Source: CAD feature listing. Evaluate the final solid. Frame: model axes, mm. Face numbers are marked on the shaded views. A direction names the side the tool comes from. Give positions to 0.01 mm unless a question says otherwise; leave off trailing zeros. Loops run counter-clockwise (first coordinate to the right, second up) from the corner with the lowest first, then second, coordinate; pieces in that order, holes last. Notation, with made-up numbers: M -21.75,10.25 L -4.75,10.25 A27 cw -4.75,29.25 Z; hole C 28.5,-38 d10. An arc over 180 degrees is marked long. Answer in a Markdown table with one row per item.
```python
from build123d import *
from OCP.BRepFilletAPI import BRepFilletAPI_MakeChamfer

# Parameters (mm, degrees)
SKETCH1_W           = 45.5
SKETCH1_H           = 9.1
BOSS_EXTRUDE1_DEPTH = 7
SKETCH2_W           = 37.1
SKETCH2_H           = 2.85
CUT_EXTRUDE1_DEPTH  = 5
SKETCH3_R           = 0.8
CUT_EXTRUDE2_DEPTH  = 5
FILLET1_R           = 1
SKETCH4_W           = 0.75
SKETCH4_H           = 0.75
BOSS_EXTRUDE2_DEPTH = 6
SKETCH5_W           = 6
SKETCH5_H           = 2
BOSS_EXTRUDE3_DEPTH = 19.5
CUT_EXTRUDE3_REACH  = 33.79
SKETCH6_W           = 3.3
SKETCH6_H           = 4.4
CHAMFER1_SIZE       = 0.25
CHAMFER1_SIZE2      = 3.575166564


with BuildPart() as part:
    # Sketch1 → Boss-Extrude1 (new body)
    with BuildSketch(Plane(origin=(0, 0, 0), x_dir=(1, 0, 0), z_dir=(0, 1, 0))):
        Rectangle(SKETCH1_W, SKETCH1_H)
    extrude(amount=BOSS_EXTRUDE1_DEPTH)

    # Sketch2 → Cut-Extrude1 (cut)
    with BuildSketch(Plane(origin=(0, 7, 0), x_dir=(1, 0, 0), z_dir=(0, 1, 0))):
        Rectangle(SKETCH2_W, SKETCH2_H)
    extrude(amount=-CUT_EXTRUDE1_DEPTH, mode=Mode.SUBTRACT)

    # Sketch3 → Cut-Extrude2 (cut)
    with BuildSketch(Plane(origin=(0, 7, 0), x_dir=(1, 0, 0), z_dir=(0, 1, 0))):
        with Locations(Location((-20.65, 0, 0), (0, 0, 270))):
            Circle(SKETCH3_R)
    extrude(amount=-CUT_EXTRUDE2_DEPTH, mode=Mode.SUBTRACT)

    # Fillet1
    fillet1_edges = [part.edges().sort_by_distance(p)[0] for p in [
        (-22.75, 7, 0),
        (0, 7, 4.55),
        (22.75, 7, 0),
        (0, 7, -4.55),
    ]]
    fillet(fillet1_edges, radius=FILLET1_R)

    # Sketch4 → Boss-Extrude2 (add)
    with BuildSketch(Plane.XZ):
        with Locations((-21.75, 2.73)):
            Rectangle(SKETCH4_W, SKETCH4_H)
        with Locations((-21.75, 0.91)):
            Rectangle(SKETCH4_W, SKETCH4_H)
        with Locations((-21.75, -0.91)):
            Rectangle(SKETCH4_W, SKETCH4_H)
        with Locations((-21.75, -2.73)):
            Rectangle(SKETCH4_W, SKETCH4_H)
    boss_extrude2 = extrude(amount=BOSS_EXTRUDE2_DEPTH)

    # Mirror1: Boss-Extrude2 across plane
    add(boss_extrude2.mirror(Plane(origin=(0, 0, 0), x_dir=(0, 0, 1), z_dir=(1, 0, 0))))

    # Sketch5 → Boss-Extrude3 (add)
    with BuildSketch(Plane(origin=(0, 2, 0), x_dir=(1, 0, 0), z_dir=(0, 1, 0))):
        Rectangle(SKETCH5_W, SKETCH5_H)
    extrude(amount=BOSS_EXTRUDE3_DEPTH)

    # Sketch6 → Cut-Extrude3 (cut, up to next)
    with BuildSketch(Plane.XY.offset(1), mode=Mode.PRIVATE) as cut_extrude3_sk1:
        with Locations((0, 19.3)):
            Rectangle(SKETCH6_W, SKETCH6_H)
    cut_extrude3_tool1 = extrude(cut_extrude3_sk1.sketch, amount=-CUT_EXTRUDE3_REACH, mode=Mode.PRIVATE) & part.part
    add(cut_extrude3_tool1.solids().sort_by_distance((0, 19.3, 1))[0], mode=Mode.SUBTRACT)

    # Chamfer1: one chamfer whose edges measure the first distance from different faces: ONE call of the kernel's chamfer builder (chamfer() names one face for all edges)
    chamfer1_edges_1 = [part.edges().sort_by_distance(p)[0] for p in [
        (-3, 21.5, 0),
    ]]
    chamfer1_side_1 = [part.faces().sort_by_distance(p)[0] for p in [
        (-2.325, 21.5, 0),
    ]]
    chamfer1_edges_2 = [part.edges().sort_by_distance(p)[0] for p in [
        (3, 21.5, 0),
    ]]
    chamfer1_side_2 = [part.faces().sort_by_distance(p)[0] for p in [
        (2.325, 21.5, 0),
    ]]
    chamfer1 = BRepFilletAPI_MakeChamfer(part.part.solid().wrapped)
    for e in chamfer1_edges_1:
        chamfer1.Add(CHAMFER1_SIZE, CHAMFER1_SIZE2, e.wrapped, chamfer1_side_1[0].wrapped)  # the first distance lies on this face
    for e in chamfer1_edges_2:
        chamfer1.Add(CHAMFER1_SIZE, CHAMFER1_SIZE2, e.wrapped, chamfer1_side_2[0].wrapped)  # the first distance lies on this face
    add(Compound.cast(chamfer1.Shape()), mode=Mode.REPLACE)


solid = part.part
```
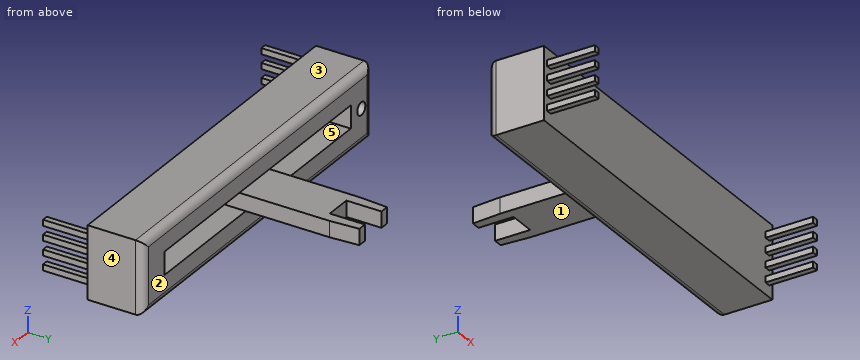
Q1. Reachability of the marked faces 4 and 5 from +Z, -Z, +X, -X, +Y, -Y: full face, straight path, thin tool, end or side. Return the list, or none.
Values follow:
| item | result |
|---|---|
| face 4 | +Z, -Z, +X, +Y, -Y |
| face 5 | +Y |
Q2. Mould query, pull axis Z, two halves, no side actions, for the marked faces 1, 2 and 3. Classes: +Z half, -Z half, draft (parallel to the pull), parting line (faces both ways), or undercut.
Values follow:
| item | result |
|---|---|
| face 1 | undercut |
| face 2 | draft |
| face 3 | +Z half |
Q3. Section query A-A (y = 5.5). Output: boundary loops of the cut face in (x, z) (3 decimals).
Values follow:
| item | result |
|---|---|
| outline | M -22.75,-4.55 L 22.75,-4.55 L 22.75,4.55 L -22.75,4.55 Z; M -3,-1 L 3,-1 L 3,1 L -3,1 Z; hole C -20.65,0 d1.6; hole M -18.55,-1.425 L 18.55,-1.425 L 18.55,1.425 L -18.55,1.425 Z |
Q4. Section query B-B (y = -3.25). Give the number of separate pieces and of enclosed holes in the cut face, plus the area to 3 significant figures.
Values follow:
| item | result |
|---|---|
| separate pieces | 8 |
| enclosed holes | 0 |
| area | 4.50 mm^2 |
Q5. Contact query for flat-ended pins moving along their axis: pin 1 Ø1.5 at (x, y) = (-1, 10) entering from +Z; pin 2 Ø4 at (x, z) = (13, -3) entering from -Y; pin 3 Ø0.8 at (y, z) = (-2, -3) entering from -X (3 decimals). Output: stop coordinate, or through.
Values follow:
| item | result |
|---|---|
| pin 1 | z = 1 |
| pin 2 | y = 0 |
| pin 3 | x = -22.125 |
Q6. Section query C-C (x = -20.65). Output: boundary loops of the cut face in (y, z).
Values follow:
| item | result |
|---|---|
| outline | M 0,-4.55 L 6,-4.55 A1 ccw 7,-3.55 L 7,-0.8 L 2,-0.8 L 2,0.8 L 7,0.8 L 7,3.55 A1 ccw 6,4.55 L 0,4.55 Z |
Q7. Section query D-D (z = 0). Output: boundary loops of the cut face in (x, y), plus the area to 3 significant figures.
Values follow:
| item | result |
|---|---|
| outline | M -22.75,0 L 22.75,0 L 22.75,6 A1 ccw 21.75,7 L 18.55,7 L 18.55,2 L 3,2 L 3,17.92 L 2.75,21.5 L 1.65,21.5 L 1.65,17.1 L -1.65,17.1 L -1.65,21.5 L -2.75,21.5 L -3,17.92 L -3,2 L -18.55,2 L -18.55,7 L -19.85,7 L -19.85,2 L -21.45,2 L -21.45,7 L -21.75,7 A1 ccw -22.75,6 Z |
| area | 226 mm^2 |
Q8. Ray query, probe 1 along X at (y, z) = (5.8, 0); probe 2 along X at (y, z) = (-0.5, 2.5) (3 decimals); probe 3 along Z at (x, y) = (-7.5, 2.5) (3 decimals). Return the intervals inside material, ascending. Write a range as from..to.
Values follow:
| item | result |
|---|---|
| probe 1 | -22.75..-21.45, -19.85..-18.55, -3..3, 18.55..22.75 |
| probe 2 | -22.125..-21.375, 21.375..22.125 |
| probe 3 | -4.55..-1.425, 1.425..4.55 |
